Input: part model. Units: mm. Frame: model coordinates. A direction names the side the tool comes from. Round coordinates to 2 decimals unless told otherwise and drop trailing zeros. Loops run counter-clockwise (first coordinate to the right, second up) from the corner with the lowest first, then second, coordinate; pieces in that order, holes last. Notation, with made-up numbers: (60, -37.75) -> (109, -37.75) arc R27 ccw to (109, -13.75) -> close; hole circle Ø11 at (-30, -40). An arc over 180 degrees is marked (long way). One line per question, with ' | ' between items. Start each with the question number.
Q1. Material intervals for L1, parallel to Z at x = 9.5, y = 7.75; L2, parallel to X at y = 1.85, z = 0; L3, parallel to Y at x = -9.5, z = 9, sorted ascending.
Q2. Contact query for flat-ended pins moving along their axis: P1, Ø6, axis at y = 6, z = -5, coming from the +X side; P2, Ø2.5, axis at x = -39.5, z = 26.5, coming from the -Y side; P3, Ø5.5, axis at y = 7, z = -26, coming from the +X side; P4, Ø1.3, axis at x = 31.5, y = 0.5, coming from the -Z side. Output: stop coordinate, or through.
Q3. Cut plane D-D on z = 21. Return loops of the section in (x, y), and give its area (3 significant figures).
Q4. Mould query, pull axis Z, two halves, no side actions, for faces 5 (the face through (22.362, 6, -26)), 6 (the face through (26.785, 1.252, -2.313)), 7 (the face through (-12.068, 3.264, 24.636)), 8 (the face through (-12, 6, 27.94)). Classes: pulls with the +Z half, pulls with the -Z half, needs draft (parallel to the pull), parting line crosses it, or undercut.
Q5. Access query for faces 1 (the face through (-37, 1, -25.4)), 2 (the face through (-44.5, 3.9, -26.4)), 3 (the face through (-12.068, 3.304, -24.676)), 4 (the face through (30, 1, -25.4)). Directions: +Z, -Z, +X, -X, +Y, -Y. A direction counts if a zero-diameter tool reaches every point of the face in a straight line with its end or side. Return the directions, or none.
Q6. Cut plane A-A on z = 0. Return loops of the section in (x, y).
Q7. Cut plane C-C on y = 11.25. Return loops of the section in (x, z).
Q8. Cut plane B-B on x = 14. Return loops of the section in (y, z).
from build123d import *

# Parameters (mm, degrees)
SKETCH1_W               = 76.2
SKETCH1_H               = 50.8
BOSS_EXTRUDE1_DEPTH     = 2.54
BOSS_EXTRUDE3_DEPTH     = 2.54
FILLET1_START           = -37.396373698
FILLET1_DEPTH           = 59.758551136
FILLET1_START_2         = -45.547043779
FILLET1_2_DEPTH         = 8.279361144
FILLET1_START_3         = 22
FILLET1_3_DEPTH         = 3.4
FILLET2_START           = -42.930825639
FILLET2_DEPTH           = 65.293003077
FILLET2_START_2         = -37.396373698
FILLET2_2_DEPTH         = 59.758551136
FILLET2_START_3         = -45.547043779
FILLET2_3_DEPTH         = 2.61621814
FILLET2_START_4         = -25.4
FILLET2_4_DEPTH         = 3.4
CUT_EXTRUDE1_DEPTH      = 74.201076537
CUT_EXTRUDE1_DEPTH_BACK = 74.201076537
SKETCH3_R               = 2.54
CUT_EXTRUDE2_DEPTH      = 55.391197925
CUT_EXTRUDE2_DEPTH_BACK = 55.391197925
SKETCH4_R               = 17.770620532


with BuildPart() as part:
    # Sketch1 → Boss-Extrude1 (new body)
    with BuildSketch(Plane(origin=(0, 0, 0), x_dir=(1, 0, 0), z_dir=(0, 1, 0))):
        Rectangle(SKETCH1_W, SKETCH1_H)
    extrude(amount=BOSS_EXTRUDE1_DEPTH)

    # Sketch2 → Boss-Extrude3 (add)
    with BuildSketch(Plane.XY.offset(25.4)):
        Polygon((22.362177438, 0), (22.362177438, 2.54), (-36.496143753, 2.54), (-33.956143753, 0), align=None)
        with BuildLine():
            Line((22.362177438, 12.7), (-31.861921757, 12.7))
            Line((-31.861921757, 12.7), (-42.930825639, 9.27384145))
            ThreePointArc((-42.930825639, 9.27384145), (-44.471302904, 8.833865445), (-45.547043679, 7.646670905))
            Line((-45.547043679, 7.646670905), (-45.547043679, 5.06740049))
            ThreePointArc((-45.547043679, 5.06740049), (-44.471302904, 3.88020595), (-42.930825639, 3.440229945))
            Line((-42.930825639, 3.440229945), (-37.396373698, 3.440229945))
            Line((-37.396373698, 3.440229945), (-36.496143753, 2.54))
            Line((-36.496143753, 2.54), (22.362177438, 2.54))
            Line((22.362177438, 2.54), (22.362177438, 12.7))
        make_face()
    boss_extrude3 = extrude(amount=BOSS_EXTRUDE3_DEPTH)

    # Fillet1: read off the stored shape, not the designer's step
    # Fillet1 outline → Fillet1 (add)
    with BuildSketch(Plane.YZ.offset(FILLET1_START)):
        with BuildLine():
            ThreePointArc((2.54, 22.86), (3.283948776, 24.656051224), (5.08, 25.4))
            Line((5.08, 25.4), (2.54, 25.4))
            Line((2.54, 25.4), (2.54, 22.86))
        make_face()
    extrude(amount=FILLET1_DEPTH)

    # Fillet1 2 outline → Fillet1 2 (add)
    with BuildSketch(Plane.YZ.offset(FILLET1_START_2)):
        with BuildLine():
            Line((3.440229945, 25.4), (3.440229945, 24.799781989))
            ThreePointArc((3.440229945, 24.799781989), (4.206915311, 25.245230204), (5.08, 25.4))
            Line((5.08, 25.4), (3.440229945, 25.4))
        make_face()
    extrude(amount=FILLET1_2_DEPTH)

    # Fillet1 3 outline → Fillet1 3 (cut)
    with BuildSketch(Plane.XY.offset(FILLET1_START_3)):
        with BuildLine():
            Line((-45.547043779, 3.440229945), (-42.930825639, 3.440229945))
            ThreePointArc((-42.930825639, 3.440229945), (-44.471302904, 3.88020595), (-45.547043679, 5.06740049))
            Line((-45.547043679, 5.06740049), (-45.547043779, 3.440229945))
        make_face()
        Polygon((-36.496143753, 2.54), (-37.396373698, 3.440229945), (-37.396373698, 2.54), align=None)
    extrude(amount=FILLET1_3_DEPTH, mode=Mode.SUBTRACT)

    # Mirror1: Boss-Extrude3 across plane
    add(boss_extrude3.mirror(Plane.XY))

    # Fillet2: read off the stored shape, not the designer's step
    # Fillet2 outline → Fillet2 (add)
    with BuildSketch(Plane.YZ.offset(FILLET2_START)):
        with BuildLine():
            ThreePointArc((5.08, -25.4), (4.206915311, -25.245230204), (3.440229945, -24.799781989))
            Line((3.440229945, -24.799781989), (3.440229945, -25.4))
            Line((3.440229945, -25.4), (5.08, -25.4))
        make_face()
    extrude(amount=FILLET2_DEPTH)

    # Fillet2 2 outline → Fillet2 2 (add)
    with BuildSketch(Plane.YZ.offset(FILLET2_START_2)):
        with BuildLine():
            ThreePointArc((3.440229945, -24.799781989), (2.776023444, -23.929248348), (2.54, -22.86))
            Line((2.54, -22.86), (2.54, -25.4))
            Line((2.54, -25.4), (3.440229945, -25.4))
            Line((3.440229945, -25.4), (3.440229945, -24.799781989))
        make_face()
    extrude(amount=FILLET2_2_DEPTH)

    # Fillet2 3 outline → Fillet2 3 (add)
    with BuildSketch(Plane.YZ.offset(FILLET2_START_3)):
        with BuildLine():
            ThreePointArc((5.08, -25.4), (4.206915311, -25.245230204), (3.440229945, -24.799781989))
            Line((3.440229945, -24.799781989), (3.440229945, -25.4))
            Line((3.440229945, -25.4), (5.08, -25.4))
        make_face()
    extrude(amount=FILLET2_3_DEPTH)

    # Fillet2 4 outline → Fillet2 4 (cut)
    with BuildSketch(Plane.XY.offset(FILLET2_START_4)):
        Polygon((-36.496143753, 2.54), (-37.396373698, 3.440229945), (-37.396373698, 2.54), align=None)
        with BuildLine():
            ThreePointArc((-42.930825639, 3.440229945), (-44.471302904, 3.88020595), (-45.547043679, 5.06740049))
            Line((-45.547043679, 5.06740049), (-45.547043779, 3.440229945))
            Line((-45.547043779, 3.440229945), (-42.930825639, 3.440229945))
        make_face()
    extrude(amount=FILLET2_4_DEPTH, mode=Mode.SUBTRACT)

    # Sketch3 → Cut-Extrude1 (cut, two sides: drawn at the far end of the back side and taken through both)
    with BuildSketch(Plane.XY.offset(27.94).offset(-CUT_EXTRUDE1_DEPTH_BACK)):
        with Locations((-22.524221352, 7.006792996)):
            Circle(SKETCH3_R)
    extrude(amount=CUT_EXTRUDE1_DEPTH + CUT_EXTRUDE1_DEPTH_BACK, mode=Mode.SUBTRACT)

    # Sketch4 → Cut-Extrude2 (cut, two sides: drawn at the far end of the back side and taken through both)
    with BuildSketch(Plane(origin=(0, 2.54, 0), x_dir=(1, 0, 0), z_dir=(0, 1, 0)).offset(-CUT_EXTRUDE2_DEPTH_BACK)):
        with Locations(Location((9.166040708, 0, 0), (0, 0, 270))):
            Circle(SKETCH4_R)
    extrude(amount=CUT_EXTRUDE2_DEPTH + CUT_EXTRUDE2_DEPTH_BACK, mode=Mode.SUBTRACT)


solid = part.part
Results:
1) L1: -27.94 to -25.4, 25.4 to 27.94 | L2: -38.1 to -8.6, 26.94 to 38.1 | L3: 0 to 2.54
2) P1: through | P2: y = 3.44 | P3: x = 22.36 | P4: z = -25.4
3) outline: (-38.1, 0) -> (38.1, 0) -> (38.1, 2.54) -> (-38.1, 2.54) -> close | area: 194 mm^2
4) face 5: needs draft | face 6: undercut | face 7: undercut | face 8: pulls with the +Z half
5) face 1: -Z, -X, -Y | face 2: +Z, -Z, -X, -Y | face 3: +X, -X, +Y | face 4: -Z, +X, +Y, -Y
6) outline: (-38.1, 0) -> (-8.6, 0) -> (-8.6, 2.54) -> (-38.1, 2.54) -> close; (26.94, 0) -> (38.1, 0) -> (38.1, 2.54) -> (26.94, 2.54) -> close
7) outline: (-36.55, -27.94) -> (22.36, -27.94) -> (22.36, -25.4) -> (-36.55, -25.4) -> close; (-36.55, 25.4) -> (22.36, 25.4) -> (22.36, 27.94) -> (-36.55, 27.94) -> close
8) outline: (0, -27.94) -> (12.7, -27.94) -> (12.7, -25.4) -> (5.08, -25.4) arc R2.54 cw to (2.54, -22.86) -> (2.54, -17.1) -> (0, -17.1) -> close; (0, 17.1) -> (2.54, 17.1) -> (2.54, 22.86) arc R2.54 cw to (5.08, 25.4) -> (12.7, 25.4) -> (12.7, 27.94) -> (0, 27.94) -> close
